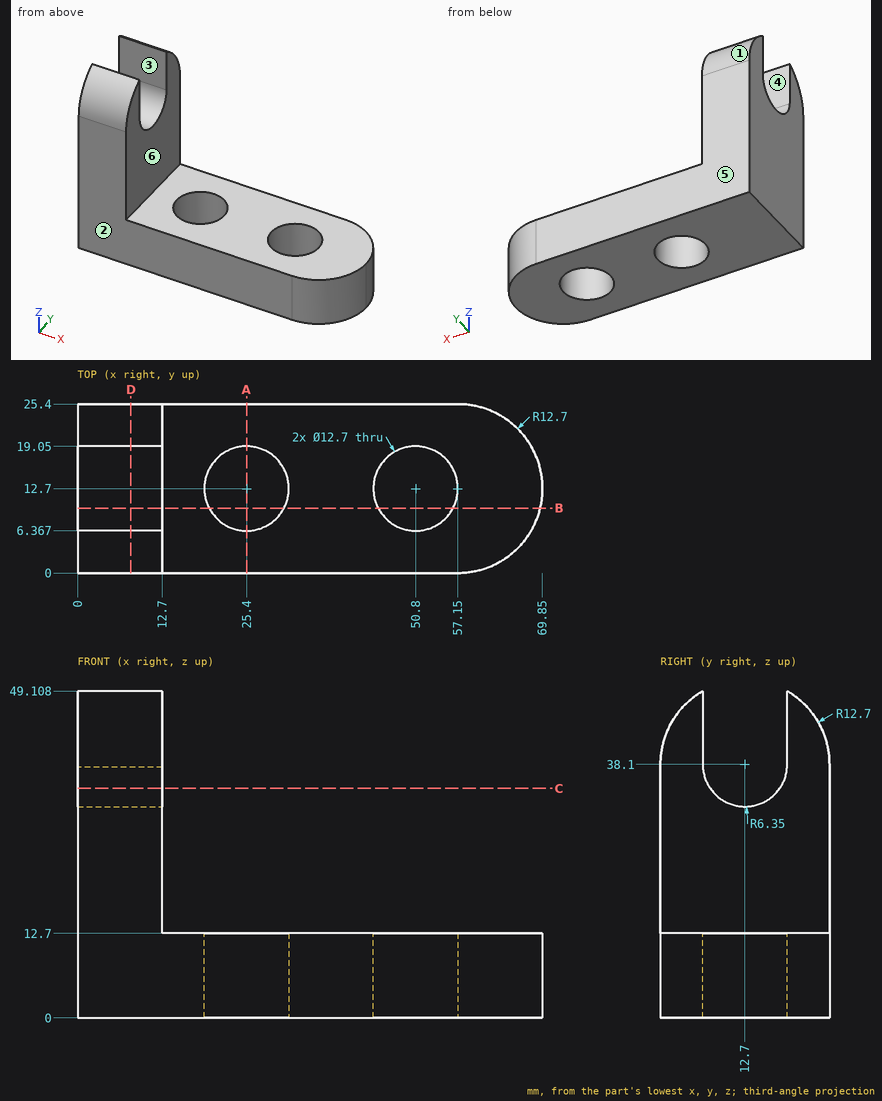
Geometry: see drawing. Coordinates: mm, zero at the bounding-box minimum. A direction names the side the tool comes from. Coordinates: 2 decimals unless noted, no trailing zeros. Loops run counter-clockwise (first coordinate to the right, second up) from the corner with the lowest first, then second, coordinate; pieces in that order, holes last.
(1) Set-up query: the marked faces 4, 5 and 6. Return all of +Z, -Z, +X, -X, +Y, -Y with unobstructed straight access to the full face (end or side cutting, diameter ignored); none if empty.
(2) Pull-direction query (Y, two-part tool) for the marked faces 1, 2 and 3; classes: released by +Y, released by -Y, zero draft, split by the parting line, or undercut.
(3) Section D-D on x = 8. Return the cut outline in (y, z).
(4) Material intervals for probe 1 along X at (y, z) = (12.75, 12.5); probe 2 along Y at (x, z) = (25.4, 9.75); probe 3 along Z at (x, y) = (55, 21), sorted ascending.
(5) First-contact query: pin 1 Ø6 at (y, z) = (12, 38.5) entering from -X; pin 2 Ø12.5 at (y, z) = (12.5, 33.5) entering from +X; pin 3 Ø9 at (x, z) = (8.5, 43.5) entering from +Y; pin 4 Ø1 at (x, y) = (34, 21) entering from +Z. Flat tips, straight axial feed; report the tip coordinate or a pass-through.
(6) Section A-A on x = 25.4. Return the cut outline in (y, z).
(7) Section C-C on z = 34.5. Return the cut outline in (x, y).
(8) Section B-B on y = 9.75. Return the cut outline in (x, z).
Data:
1. face 4: +Z, +X, -X
1. face 5: +Z, -Z, +X, -X, +Y
1. face 6: +Z, +X, +Y, -Y
2. face 1: released by +Y
2. face 2: released by -Y
2. face 3: undercut
3. outline: (0, 0) - (25.4, 0) - (25.4, 38.1) arc R12.7 ccw to (19.05, 49.1) - (19.05, 38.1) arc R6.35 cw to (6.37, 37.64) - (6.37, 49.11) arc R12.7 ccw to (0, 38.1) - close
4. probe 1: x = 0 to 19.05, 31.75 to 44.45, 57.15 to 69.85
4. probe 2: y = 0 to 6.35, 19.05 to 25.4
4. probe 3: z = 0 to 12.7
5. pin 1: passes through
5. pin 2: stops at x = 12.7
5. pin 3: stops at y = 25.37
5. pin 4: stops at z = 12.7
6. outline: (0, 0) - (6.35, 0) - (6.35, 12.7) - (0, 12.7) - close; (19.05, 0) - (25.4, 0) - (25.4, 12.7) - (19.05, 12.7) - close
7. outline: (0, 0) - (12.7, 0) - (12.7, 7.47) - (0, 7.47) - close; (0, 17.93) - (12.7, 17.93) - (12.7, 25.4) - (0, 25.4) - close
8. outline: (0, 0) - (19.78, 0) - (19.78, 12.7) - (12.7, 12.7) - (12.7, 32.48) - (0, 32.48) - close; (31.02, 0) - (45.18, 0) - (45.18, 12.7) - (31.02, 12.7) - close; (56.42, 0) - (69.5, 0) - (69.5, 12.7) - (56.42, 12.7) - close
